```python
from build123d import *

# Parameters (mm, degrees)
ESBO_O1_W                = 6
ESBO_O1_H                = 65
RESSALTO_EXTRUS_O1_DEPTH = 21
RESSALTO_EXTRUS_O4_DEPTH = 5
CORTE_EXTRUS_O6_START    = -1
CORTE_EXTRUS_O6_DEPTH    = 4
CHANFRO1_SIZE            = 6.4
CHANFRO2_SIZE            = 6.4
ESBO_O15_R               = 1.65
CORTE_EXTRUS_O7_DEPTH    = 41.227478171
CORTE_EXTRUS_O8_DEPTH    = 2
ESBO_O17_R               = 3.5
CORTE_EXTRUS_O9_DEPTH    = 2.5
CORTE_EXTRUS_O10_DEPTH   = 40.15673633


with BuildPart() as part:
    # Esboço1 → Ressalto-extrusão1 (new, symmetric)
    with BuildSketch(Plane.XY):
        with Locations((3, 0)):
            Rectangle(ESBO_O1_W, ESBO_O1_H)
    extrude(amount=RESSALTO_EXTRUS_O1_DEPTH, both=True)

    # Esboço11 → Ressalto-extrusão4 (add)
    with BuildSketch(Plane.ZY):
        Polygon((-17.5, -9.5), (0, -16.5), (17.5, -9.5), (17.5, 23.5), (21, 23.5), (21, -16.716263691), (0, -25.116263691), (-21, -16.716263691), (-21, 23.5), (-17.5, 23.5), align=None)
    extrude(amount=RESSALTO_EXTRUS_O4_DEPTH)

    # Esboço12 → Corte-extrusão6 (cut)
    with BuildSketch(Plane.ZY.offset(5).offset(CORTE_EXTRUS_O6_START)):
        Polygon((-17.5, -9.5), (17.5, -9.5), (17.5, -16.5), (0, -23.5), (-17.5, -16.5), align=None)
    extrude(amount=-CORTE_EXTRUS_O6_DEPTH, mode=Mode.SUBTRACT)

    # Chanfro1
    # the kernel refuses this chamfer: 6.4 mm, written as the material it adds along each edge
    with BuildSketch(Plane(origin=(-4, -29.612634139, 15.281585348), x_dir=(-0.0274958766105864, 0.9281256495501803, 0.3712502598200724), z_dir=(0, 0.371390676354104, -0.9284766908852593))) as chanfro1_piece_1_section:
        Polygon((CHANFRO1_SIZE * 0.999621916911, CHANFRO1_SIZE * 0.0274958766106), (-CHANFRO1_SIZE * 0.0274958766106, CHANFRO1_SIZE * 0.999621916911), (0, 0), align=None)
    chanfro1_piece_1 = extrude(amount=51.765619071, mode=Mode.PRIVATE)
    chanfro1_piece_1 = split(chanfro1_piece_1, bisect_by=Plane(origin=(-1.981352532, -18.155988855, -17.5), z_dir=(0, 0, 1)), keep=Keep.TOP, mode=Mode.PRIVATE)
    chanfro1_piece_1 = split(chanfro1_piece_1, bisect_by=Plane(origin=(-1.981352532, -25.250248134, -4.375620334), z_dir=(0, 0.9284766908852594, -0.3713906763541037)), keep=Keep.TOP, mode=Mode.PRIVATE)
    add(chanfro1_piece_1)
    with BuildSketch(Plane(origin=(-4, -10.387365861, 32.781585348), x_dir=(-0.027495876610586396, 0.9281256495501804, -0.37125025982007215), z_dir=(0, -0.3713906763541037, -0.9284766908852594))) as chanfro1_piece_2_section:
        Polygon((CHANFRO1_SIZE * 0.999621916911, CHANFRO1_SIZE * 0.0274958766106), (-CHANFRO1_SIZE * 0.0274958766106, CHANFRO1_SIZE * 0.999621916911), (0, 0), align=None)
    chanfro1_piece_2 = extrude(amount=51.765619071, mode=Mode.PRIVATE)
    chanfro1_piece_2 = split(chanfro1_piece_2, bisect_by=Plane(origin=(-1.981352532, -18.155988855, 17.5), z_dir=(0, 0, -1)), keep=Keep.TOP, mode=Mode.PRIVATE)
    chanfro1_piece_2 = split(chanfro1_piece_2, bisect_by=Plane(origin=(-1.981352532, -25.250248134, 4.375620334), z_dir=(0, 0.9284766908852593, 0.371390676354104)), keep=Keep.TOP, mode=Mode.PRIVATE)
    add(chanfro1_piece_2)

    # Chanfro2
    # the kernel refuses this chamfer: 6.4 mm, written as the material it adds along each edge
    with BuildSketch(Plane(origin=(0, -31.228897831, 15.281585348), x_dir=(-0.9996219169112968, 0.025529280528386766, 0.010211712211354711), z_dir=(0, 0.37139067635410383, -0.9284766908852593))) as chanfro2_piece_1_section:
        Polygon((CHANFRO2_SIZE * 0.999621916911, -CHANFRO2_SIZE * 0.0274958766106), (-CHANFRO2_SIZE * 0.0274958766106, -CHANFRO2_SIZE * 0.999621916911), (0, 0), align=None)
    chanfro2_piece_1 = extrude(amount=55.535234436, mode=Mode.PRIVATE)
    chanfro2_piece_1 = split(chanfro2_piece_1, bisect_by=Plane(origin=(-5, -22.562055234, -11.871492952), z_dir=(1, 0, 0)), keep=Keep.TOP, mode=Mode.PRIVATE)
    chanfro2_piece_1 = split(chanfro2_piece_1, bisect_by=Plane(origin=(-1.967131821, -22.562055234, -21), z_dir=(0, 0, 1)), keep=Keep.TOP, mode=Mode.PRIVATE)
    chanfro2_piece_1 = split(chanfro2_piece_1, bisect_by=Plane(origin=(-1.967131821, -28.857577336, -9.353284111), z_dir=(0, 0.9284766908852593, -0.37139067635410383)), keep=Keep.TOP, mode=Mode.PRIVATE)
    add(chanfro2_piece_1)
    with BuildSketch(Plane(origin=(0, -10.603629552, 36.281585348), x_dir=(-0.9996219169112968, 0.02552928052838644, -0.010211712211354581), z_dir=(0, -0.37139067635410383, -0.9284766908852593))) as chanfro2_piece_2_section:
        Polygon((CHANFRO2_SIZE * 0.999621916911, -CHANFRO2_SIZE * 0.0274958766106), (-CHANFRO2_SIZE * 0.0274958766106, -CHANFRO2_SIZE * 0.999621916911), (0, 0), align=None)
    chanfro2_piece_2 = extrude(amount=55.535234436, mode=Mode.PRIVATE)
    chanfro2_piece_2 = split(chanfro2_piece_2, bisect_by=Plane(origin=(-5, -22.562055234, 11.871492952), z_dir=(1, 0, 0)), keep=Keep.TOP, mode=Mode.PRIVATE)
    chanfro2_piece_2 = split(chanfro2_piece_2, bisect_by=Plane(origin=(-1.967131821, -22.562055234, 21), z_dir=(0, 0, -1)), keep=Keep.TOP, mode=Mode.PRIVATE)
    chanfro2_piece_2 = split(chanfro2_piece_2, bisect_by=Plane(origin=(-1.967131821, -28.857577336, 9.353284111), z_dir=(0, 0.9284766908852593, 0.37139067635410383)), keep=Keep.TOP, mode=Mode.PRIVATE)
    add(chanfro2_piece_2)
    with BuildSketch(Plane(origin=(0, -10.603629552, 36.281585348), x_dir=(-0.9996219169112968, 0.02552928052838644, -0.010211712211354581), z_dir=(0, -0.37139067635410383, -0.9284766908852593))) as chanfro2_piece_3a_section:
        Polygon((CHANFRO2_SIZE * 0.999621916911, -CHANFRO2_SIZE * 0.0274958766106), (-CHANFRO2_SIZE * 0.0274958766106, -CHANFRO2_SIZE * 0.999621916911), (0, 0), align=None)
    chanfro2_piece_3a = extrude(amount=55.535234436, mode=Mode.PRIVATE)
    chanfro2_piece_3a = split(chanfro2_piece_3a, bisect_by=Plane(origin=(-5, -29.234460618, -4.706755421), z_dir=(1, 0, 0)), keep=Keep.TOP, mode=Mode.PRIVATE)
    chanfro2_piece_3a = split(chanfro2_piece_3a, bisect_by=Plane(origin=(-1.958615866, -24.061271743, -2.637479871), z_dir=(0, -0.9284766908852593, -0.37139067635410383)), keep=Keep.TOP, mode=Mode.PRIVATE)
    chanfro2_piece_3a = split(chanfro2_piece_3a, bisect_by=Plane(origin=(-1.958615866, -32.5, -4.706755421), z_dir=(0, 1, 0)), keep=Keep.TOP, mode=Mode.PRIVATE)
    with BuildSketch(Plane(origin=(0, -31.228897831, 15.281585348), x_dir=(-0.9996219169112968, 0.025529280528386766, 0.010211712211354711), z_dir=(0, 0.37139067635410383, -0.9284766908852593))) as chanfro2_piece_3b_section:
        Polygon((CHANFRO2_SIZE * 0.999621916911, -CHANFRO2_SIZE * 0.0274958766106), (-CHANFRO2_SIZE * 0.0274958766106, -CHANFRO2_SIZE * 0.999621916911), (0, 0), align=None)
    chanfro2_piece_3b = extrude(amount=55.535234436, mode=Mode.PRIVATE)
    chanfro2_piece_3b = split(chanfro2_piece_3b, bisect_by=Plane(origin=(-5, -29.234460618, 4.706755421), z_dir=(1, 0, 0)), keep=Keep.TOP, mode=Mode.PRIVATE)
    chanfro2_piece_3b = split(chanfro2_piece_3b, bisect_by=Plane(origin=(-1.958615866, -24.061271743, 2.637479871), z_dir=(0, -0.9284766908852593, 0.37139067635410383)), keep=Keep.TOP, mode=Mode.PRIVATE)
    chanfro2_piece_3b = split(chanfro2_piece_3b, bisect_by=Plane(origin=(-1.958615866, -32.5, 4.706755421), z_dir=(0, 1, 0)), keep=Keep.TOP, mode=Mode.PRIVATE)
    chanfro2_piece_3 = chanfro2_piece_3a & chanfro2_piece_3b
    add(chanfro2_piece_3)

    # Esboço15 → Corte-extrusão7 (cut, through all)
    with BuildSketch(Plane.ZY.offset(5)):
        with Locations((0, 28)):
            Circle(ESBO_O15_R)
        with Locations((0, 20.5)):
            Circle(ESBO_O15_R)
        with Locations((0, -9.5)):
            Circle(ESBO_O15_R)
    extrude(amount=-CORTE_EXTRUS_O7_DEPTH, mode=Mode.SUBTRACT)

    # Esboço16 → Corte-extrusão8 (cut)
    with BuildSketch(Plane(origin=(6, 0, 0), x_dir=(0, 0, -1), z_dir=(1, 0, 0))):
        Polygon((3.233161507, 28), (1.616580754, 30.8), (-1.616580754, 30.8), (-3.233161507, 28), (-1.616580754, 25.2), (1.616580754, 25.2), align=None)
    extrude(amount=-CORTE_EXTRUS_O8_DEPTH, mode=Mode.SUBTRACT)

    # Esboço17 → Corte-extrusão9 (cut)
    with BuildSketch(Plane.ZY):
        with Locations((0, 20.5)):
            Circle(ESBO_O17_R)
        with Locations((0, -9.5)):
            Circle(ESBO_O17_R)
    extrude(amount=-CORTE_EXTRUS_O9_DEPTH, mode=Mode.SUBTRACT)

    # Esboço18 → Corte-extrusão10 (cut, through all)
    with BuildSketch(Plane.ZY):
        Polygon((21, -23.609274645), (0, -32.009274645), (-21, -23.609274645), (-21, -32.5), (21, -32.5), align=None)
    extrude(amount=-CORTE_EXTRUS_O10_DEPTH, mode=Mode.SUBTRACT)


solid = part.part
```
Geometry: final body of the model. Coordinates: model frame, mm. A direction names the side the tool comes from. Round coordinates to 2 decimals unless told otherwise and drop trailing zeros. Loops run counter-clockwise (first coordinate to the right, second up) from the corner with the lowest first, then second, coordinate; pieces in that order, holes last.
Item 1: Section D-D, the plane z = 7.5. Output: boundary loops of the cut face in (x, y), plus the area to 3 significant figures.
Checked values:
outline: (-5, -23.62) - (0, -29.01) - (6, -29.01) - (6, 32.5) - (0, 32.5) - (0, -17.92) - (-4, -13.61) - (-4, -13.5) - (-5, -13.5) - close
area: 424 mm2
Item 2: Mould query, pull axis Y, two halves, no side actions, for faces 1 (the flat face through (5.014, 26.62, 2.436)), 2 (the flat face through (-2, 5, 17.5)), 3 (the flat face through (2.96, -27.87, -10.35)). Classes: released by +Y, released by -Y, zero draft, split by the parting line, or undercut.
Checked values:
face 1: undercut
face 2: zero draft
face 3: released by -Y
Item 3: Contact query for flat-ended pins moving along their axis: P1, Ø5.5, axis at y = 20.5, z = 0.5, coming from the -X side; P2, Ø5, axis at x = -3.5, z = 6, coming from the +Y side; P3, Ø8, axis at y = -9.5, z = 0, coming from the -X side; P4, Ø1.7, axis at y = 28.5, z = 0, coming from the +X side. Output: stop coordinate, or through.
Checked values:
P1: stops at x = 2.5
P2: stops at y = -13.12
P3: stops at x = 0
P4: passes through
Item 4: Section B-B, the plane y = 20.5. Output: boundary loops of the cut face in (x, z).
Checked values:
outline: (-5, -21) - (6, -21) - (6, -1.65) - (2.5, -1.65) - (2.5, -3.5) - (0, -3.5) - (0, -17.5) - (-5, -17.5) - close; (-5, 17.5) - (0, 17.5) - (0, 3.5) - (2.5, 3.5) - (2.5, 1.65) - (6, 1.65) - (6, 21) - (-5, 21) - close
Item 5: Section A-A, the plane x = 1.5. Output: boundary loops of the cut face in (y, z), plus the area to 3 significant figures.
Checked values:
outline: (-32.01, 0) - (-23.61, -21) - (32.5, -21) - (32.5, 21) - (-23.61, 21) - close; hole circle Ø7 at (-9.5, 0); hole circle Ø7 at (20.5, 0); hole circle Ø3.3 at (28, 0)
area: 2,450 mm2
Item 6: Section C-C, the plane y = 6.5. Output: boundary loops of the cut face in (x, z).
Checked values:
outline: (-5, -21) - (6, -21) - (6, 21) - (-5, 21) - (-5, 17.5) - (0, 17.5) - (0, -17.5) - (-5, -17.5) - close
Item 7: Reachability of faces 4 (the flat face through (-4.49, -12.95, -8.87)), 5 (the flat face through (6, 0, 0)), 6 (the flat face through (5.014, 29.38, -2.436)), 7 (the flat face through (0, 5, -21)), 8 (the flat face through (2.5, -11, 1)) from +Z, -Z, +X, -X, +Y, -Y: full face, straight path, thin tool, end or side. Return the list, or none.
Checked values:
face 4: -X, +Y
face 5: +Z, -Z, +X, +Y, -Y
face 6: +X
face 7: -Z, +X, -X, +Y, -Y
face 8: -X
Item 8: Line query: L1, parallel to Y at x = 3.7, z = 0; L2, parallel to Y at x = 4.7, z = 0; L3, parallel to Z at x = -0.5, y = -6. Output: solid intervals per line, ascending.
Checked values:
L1: y = -32.01 to -11.15, -7.85 to 18.85, 22.15 to 26.35, 29.65 to 32.5
L2: y = -32.01 to -11.15, -7.85 to 18.85, 22.15 to 25.2, 30.8 to 32.5
L3: z = -21 to -17.5, 17.5 to 21
